CAD build for the part. Positions are in the model's coordinates, mm. Face numbers are marked on the shaded views. Give positions to 0.01 mm unless a question says otherwise; leave off trailing zeros. Write each loop counter-clockwise with the first axis right and the second up, starting at its lowest first coordinate (ties: lowest second). Pieces come first, ordered by that corner, then holes. Notation, with made-up numbers: (73.5, -15.75) -> (85.5, -15.75) arc R16 ccw to (85.5, -5.75) -> close; hole circle Ø1 at (11, -35). An arc over 180 degrees is marked (long way). Answer in a Markdown table with one row per item. Add a question column.
```python
from build123d import *

# Parameters (mm, degrees)
SKETCH1_R           = 2.5
SKETCH1_R_2         = 1.5
SKETCH1_R_3         = 1.65
BOSS_EXTRUDE1_DEPTH = 4.15


with BuildPart() as part:
    # Sketch1 → Boss-Extrude1 (new body)
    with BuildSketch(Plane(origin=(0, -205, 0), x_dir=(1, 0, 0), z_dir=(0, 1, 0))):
        Polygon((52, 38.5), (64, 50), (95, 50), (102.5, 43), (102.5, 17), (92.5, 0), (-92.5, 0), (-102.5, 17), (-102.5, 43), (-95, 50), (-64, 50), (-52, 38.5), align=None)
        with Locations(Location((-96.6, 40.1, 0), (0, 0, 270))):  # turned: the seam where the file's is
            Circle(SKETCH1_R, mode=Mode.SUBTRACT)
        with Locations(Location((-73.4, 40.1, 0), (0, 0, 270))):  # turned: the seam where the file's is
            Circle(SKETCH1_R, mode=Mode.SUBTRACT)
        with Locations(Location((-96.6, 16.9, 0), (0, 0, 270))):  # turned: the seam where the file's is
            Circle(SKETCH1_R, mode=Mode.SUBTRACT)
        with Locations(Location((-73.4, 16.9, 0), (0, 0, 270))):  # turned: the seam where the file's is
            Circle(SKETCH1_R, mode=Mode.SUBTRACT)
        with Locations(Location((-90.5, 10, 0), (0, 0, 270))):  # turned: the seam where the file's is
            Circle(SKETCH1_R_2, mode=Mode.SUBTRACT)
        with Locations(Location((-79.5, 10, 0), (0, 0, 270))):  # turned: the seam where the file's is
            Circle(SKETCH1_R_2, mode=Mode.SUBTRACT)
        with Locations(Location((-60, 29, 0), (0, 0, 270))):  # turned: the seam where the file's is
            Circle(SKETCH1_R_3, mode=Mode.SUBTRACT)
        with Locations(Location((-60, 18, 0), (0, 0, 270))):  # turned: the seam where the file's is
            Circle(SKETCH1_R_3, mode=Mode.SUBTRACT)
        with Locations(Location((0, 30, 0), (0, 0, 270))):  # turned: the seam where the file's is
            Circle(SKETCH1_R_2, mode=Mode.SUBTRACT)
        with Locations(Location((0, 4, 0), (0, 0, 270))):  # turned: the seam where the file's is
            Circle(SKETCH1_R_2, mode=Mode.SUBTRACT)
        with Locations(Location((73.4, 40.1, 0), (0, 0, 90))):  # turned: the seam where the file's is
            Circle(SKETCH1_R, mode=Mode.SUBTRACT)
        with Locations(Location((60, 29, 0), (0, 0, 90))):  # turned: the seam where the file's is
            Circle(SKETCH1_R_3, mode=Mode.SUBTRACT)
        with Locations(Location((60, 18, 0), (0, 0, 90))):  # turned: the seam where the file's is
            Circle(SKETCH1_R_3, mode=Mode.SUBTRACT)
        with Locations(Location((73.4, 16.9, 0), (0, 0, 90))):  # turned: the seam where the file's is
            Circle(SKETCH1_R, mode=Mode.SUBTRACT)
        with Locations(Location((79.5, 10, 0), (0, 0, 90))):  # turned: the seam where the file's is
            Circle(SKETCH1_R_2, mode=Mode.SUBTRACT)
        with Locations(Location((90.5, 10, 0), (0, 0, 90))):  # turned: the seam where the file's is
            Circle(SKETCH1_R_2, mode=Mode.SUBTRACT)
        with Locations(Location((96.6, 16.9, 0), (0, 0, 90))):  # turned: the seam where the file's is
            Circle(SKETCH1_R, mode=Mode.SUBTRACT)
        with Locations(Location((96.6, 40.1, 0), (0, 0, 90))):  # turned: the seam where the file's is
            Circle(SKETCH1_R, mode=Mode.SUBTRACT)
    extrude(amount=-BOSS_EXTRUDE1_DEPTH)


solid = part.part
```
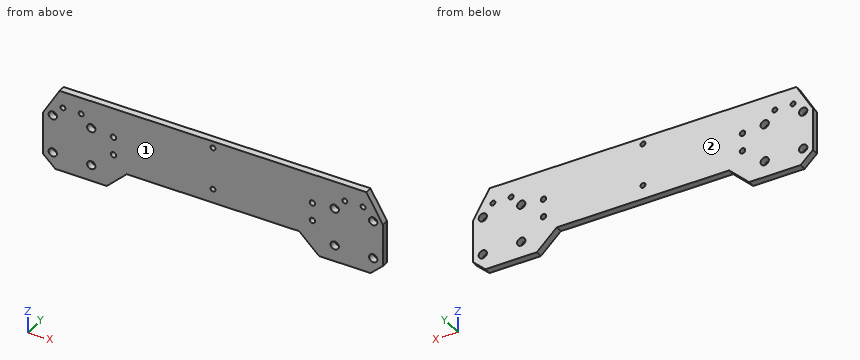
Item 1: Slice it at C-C, the plane z = -45. List the corners of the cut face in (x, y).
Item 2: Probe L1, parallel to X at y = -206.9, z = -40.1; L2, parallel to Z at x = 18.5, y = -206.85; L3, parallel to X at y = -208, z = -29. List the from-to ranges inside material, lowest first. Write a range as from..to.
Item 3: Slice it at D-D, the plane x = -8. List the corners of the cut face in (y, z).
Item 4: Slice it at B-B, the plane y = -207.05. State how many separate pieces and enclosed holes the cut face has, then the cut area to 3 significant figures.
Item 5: Mould opens along Y. For the marked faces 1 and 2 say: released by +Y, released by -Y, zero draft, split by the parting line, or undercut.
Item 6: Drop flat-ended pins along their axis: pin 1 Ø4.5 at (x, z) = (73.4, -16.9) entering from -Y; pin 2 Ø1.5 at (y, z) = (-206, -16) entering from +X; pin 3 Ø2 at (x, y) = (8.5, -206) entering from -Z. Give the stop position or say it passes through.
Item 7: Slice it at A-A, the plane x = 73.4. List the corners of the cut face in (y, z).
Answer key:
| question | item | result |
|---|---|---|
| 1 | outline | (-100.36, -209.15) -> (-58.78, -209.15) -> (-58.78, -205) -> (-100.36, -205) -> close; (58.78, -209.15) -> (100.36, -209.15) -> (100.36, -205) -> (58.78, -205) -> close |
| 2 | L1 | x = -102.5..-99.1, -94.1..-75.9, -70.9..-53.67, 53.67..70.9, 75.9..94.1, 99.1..102.5 |
| 2 | L2 | z = -38.5..0 |
| 2 | L3 | x = -102.5..-61.65, -58.35..-1.12, 1.12..58.35, 61.65..102.5 |
| 3 | outline | (-209.15, -38.5) -> (-205, -38.5) -> (-205, 0) -> (-209.15, 0) -> close |
| 4 | separate pieces | 1 |
| 4 | enclosed holes | 18 |
| 4 | area | 8,460 mm² |
| 5 | face 1 | released by -Y |
| 5 | face 2 | released by +Y |
| 6 | pin 1 | passes through |
| 6 | pin 2 | stops at x = 102.35 |
| 6 | pin 3 | stops at z = -38.5 |
| 7 | outline | (-209.15, -50) -> (-205, -50) -> (-205, -42.6) -> (-209.15, -42.6) -> close; (-209.15, -37.6) -> (-205, -37.6) -> (-205, -19.4) -> (-209.15, -19.4) -> close; (-209.15, -14.4) -> (-205, -14.4) -> (-205, 0) -> (-209.15, 0) -> close |
